```python
from build123d import *

# Parameters (mm, degrees)
SKETCH1_R           = 13.5
BOSS_EXTRUDE1_DEPTH = 8
BOSS_EXTRUDE3_START = 12
SKETCH7_R           = 7.5
BOSS_EXTRUDE3_DEPTH = 12
SKETCH4_W           = 28
SKETCH4_H           = 10
CUT_EXTRUDE2_DEPTH  = 12
SKETCH5_R           = 2
CUT_EXTRUDE3_DEPTH  = 100
SKETCH9_R           = 8
SKETCH9_R_2         = 2
BOSS_EXTRUDE4_DEPTH = 40
FILLET2_R           = 10
FILLET3_R           = 3
SKETCH11_R          = 8
CUT_EXTRUDE6_DEPTH  = 14


with BuildPart() as part:
    # Sketch1 → Boss-Extrude1 (new body)
    with BuildSketch(Plane(origin=(0, 0, 0), x_dir=(1, 0, 0), z_dir=(0, 1, 0))):
        with BuildLine():
            Line((2.5, -44.330127019), (37.141016151, -24.330127019))
            Line((37.141016151, -24.330127019), (29.641016151, -11.339745962))
            ThreePointArc((29.641016151, -11.339745962), (24.078586932, -9.298131712), (20, -5))
            Line((20, -5), (20, 5))
            ThreePointArc((20, 5), (15.606601718, 15.606601718), (5, 20))
            Line((5, 20), (-14, 20))
            Line((-14, 20), (-23.593165935, 30.196625292))
            Line((-23.593165935, 30.196625292), (-34.466370956, 19.863503181))
            Line((-34.466370956, 19.863503181), (-20, 4.641016151))
            Line((-20, 4.641016151), (-20, -5.358983849))
            Line((-20, -5.358983849), (2.5, -44.330127019))
        make_face()
        with Locations(Location((0, 0, 0), (0, 0, 270))):
            Circle(SKETCH1_R, mode=Mode.SUBTRACT)
    extrude(amount=BOSS_EXTRUDE1_DEPTH)

    # Sketch7 → Boss-Extrude3 (add)
    with BuildSketch(Plane.XZ.offset(BOSS_EXTRUDE3_START)):
        with BuildLine():
            Line((20, 5), (20, -5))
            ThreePointArc((20, -5), (15.606601718, -15.606601718), (5, -20))
            Line((5, -20), (-14, -20))
            Line((-14, -20), (-23.593165935, -30.196625292))
            Line((-23.593165935, -30.196625292), (-34.466370956, -19.863503181))
            Line((-34.466370956, -19.863503181), (-20, -4.641016151))
            Line((-20, -4.641016151), (-20, 5.358983849))
            Line((-20, 5.358983849), (2.5, 44.330127019))
            Line((2.5, 44.330127019), (37.141016151, 24.330127019))
            Line((37.141016151, 24.330127019), (29.641016151, 11.339745962))
            ThreePointArc((29.641016151, 11.339745962), (24.078586932, 9.298131712), (20, 5))
        make_face()
        with Locations(Location((0, 0, 0), (0, 0, 270))):
            Circle(SKETCH7_R, mode=Mode.SUBTRACT)
    extrude(amount=-BOSS_EXTRUDE3_DEPTH)

    # Sketch4 → Cut-Extrude2 (cut)
    with BuildSketch(Plane(origin=(19.820508076, 0, 34.330127019), x_dir=(0.8660254037844378, 0, -0.5000000000000016), z_dir=(0.5000000000000014, 0, 0.8660254037844377))):
        with Locations((0, -7)):
            Rectangle(SKETCH4_W, SKETCH4_H)
    extrude(amount=-CUT_EXTRUDE2_DEPTH, mode=Mode.SUBTRACT)

    # Sketch5 → Cut-Extrude3 (cut)
    with BuildSketch(Plane(origin=(17.320508076, 0, -10), x_dir=(-0.5000000000000026, 0, -0.8660254037844373), z_dir=(0.8660254037844373, 0, -0.5000000000000026))):
        with Locations((-33.641016151, -7)):
            Circle(SKETCH5_R)
    extrude(amount=-CUT_EXTRUDE3_DEPTH, mode=Mode.SUBTRACT)

    # Sketch9 → Boss-Extrude4 (add)
    with BuildSketch(Plane(origin=(17.320508076, 0, -10), x_dir=(-0.5000000000000017, 0, -0.8660254037844378), z_dir=(0.8660254037844377, 0, -0.5000000000000016))):
        with Locations((-33.641016151, -7)):
            Circle(SKETCH9_R)
        with Locations((-33.641016151, -7)):
            Circle(SKETCH9_R_2, mode=Mode.SUBTRACT)
    extrude(amount=-BOSS_EXTRUDE4_DEPTH)

    # Fillet2
    fillet2_edges = [part.edges().sort_by_distance(p)[0] for p in [
        (-20, -2, 5.358983849),
        (-20, -2, -4.641016151),
        (-14, -2, -20),
    ]]
    fillet(fillet2_edges, radius=FILLET2_R)

    # Fillet3
    fillet3_edges = [part.edges().sort_by_distance(p)[0] for p in [
        (-34.466370956, -2, -19.863503181),
        (-23.593165935, -2, -30.196625292),
    ]]
    fillet(fillet3_edges, radius=FILLET3_R)

    # Sketch11 → Cut-Extrude6 (cut, symmetric)
    with BuildSketch(Plane(origin=(0, 0, 0), x_dir=(-0.5000000000000017, 0, -0.8660254037844378), z_dir=(0.8660254037844377, 0, -0.5000000000000016))):
        with Locations((-33.641016151, -7)):
            Circle(SKETCH11_R)
    extrude(amount=CUT_EXTRUDE6_DEPTH, both=True, mode=Mode.SUBTRACT)


solid = part.part
```
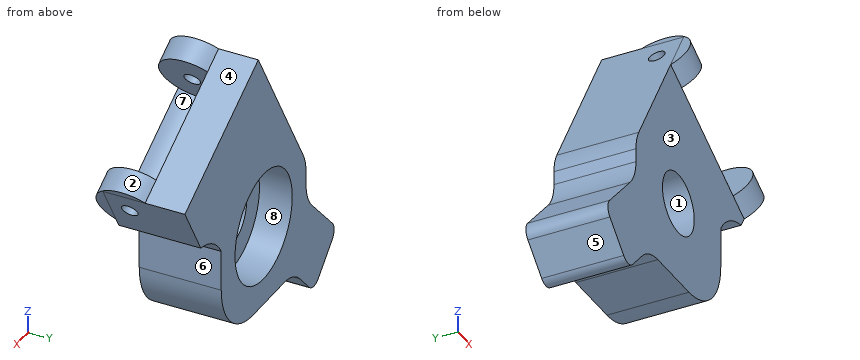
Part model, mm, in its own coordinate system. Face numbers are marked on the shaded views. A direction names the side the tool comes from. Round coordinates to 2 decimals unless told otherwise and drop trailing zeros. Write each loop counter-clockwise with the first axis right and the second up, starting at its lowest first coordinate (ties: lowest second). Pieces come first, ordered by that corner, then holes. Notation, with made-up numbers: (-30, -19.5) -> (-14, -19.5) arc R21 ccw to (-14, 17.5) -> close; hole circle Ø9 at (-19, -18). An arc over 180 degrees is marked (long way). Return JSON: item names as keys, results as strings. Group by question number.
Q1. Saw through at A-A on x = -6.5. Write the cut outline in (y, z).
Q2. Pin check, flat tips, straight feed: pin 1 (1.5 mm diameter, centred on y = 5.5, z = 31.5, fed in from -X); pin 2 (2 mm diameter, centred on y = -6, z = -16, fed in from +X); pin 3 (1 mm diameter, centred on y = -4.5, z = 0.5, fed in from -X). Stop position of each tip, or through.
Q3. Which spindle directions (+Z, -Z, +X, -X, +Y, -Y) get a long thin tool onto all of the face, cutting with end or side? Do the marked faces 4, 5, 6, 7 and 8. Say none if no direction does.
Q4. Saw through at B-B on y = -13.5. Write the cut outline in (x, z).
Q5. Probe L1, parallel to X at y = -5.75, z = 0; L2, parallel to X at y = 3.5, z = 0; L3, parallel to Y at x = -20, z = -6.5. List the from-to ranges inside material, lowest first. Write a range as [from, to].
Q6. Mould opens along X. For the marked faces 1, 2 and 3 say: pulls with the +X half, pulls with the -X half, needs draft (parallel to the pull), parting line crosses it, or undercut.
Q7. Saw through at C-C on z = -19. Write the cut outline in (x, y), plus the area to 3 significant figures.
Answer:
{
 "1": {"outline": "(-12, -20) -> (8, -20) -> (8, -11.83) -> (0, -11.83) -> (0, -3.74) -> (-12, -3.74) -> close; (-12, 3.74) -> (0, 3.74) -> (0, 11.83) -> (8, 11.83) -> (8, 28.74) -> (-12, 28.74) -> close"},
 "2": {"pin 1": "x = -5.34", "pin 2": "x = 16.18", "pin 3": "x = -20"},
 "3": {"face 4": "+Z, +X, +Y", "face 5": "-Z, -X, +Y, -Y", "face 6": "-Z, +X, +Y, -Y", "face 7": "none", "face 8": "+Y"},
 "4": {"outline": "(-2.83, 35.1) -> (2.36, 32.1) -> (7.03, 40.17) -> (1.83, 43.17) -> close; (26.61, 18.1) -> (31.81, 15.1) -> (36.47, 23.17) -> (31.28, 26.17) -> close"},
 "5": {"L1": "[-20, -7.5], [7.5, 20]", "L2": "[-20, -13.5], [13.5, 20]", "L3": "[-12, 8]"},
 "6": {"face 1": "undercut", "face 2": "parting line crosses it", "face 3": "needs draft"},
 "7": {"outline": "(-33.13, -12) -> (10.39, -12) -> (10.39, 8) -> (-33.13, 8) -> close", "area": "870 mm2"}
}
